Here's how the part is built. I have some questions about the finished solid (model axes, mm). Round coordinates to 2 decimals unless told otherwise and drop trailing zeros. Order: outer loops, then holes, each group sorted by start corner. A loop starts at its lowest first (then second) coordinate and runs counter-clockwise, first axis right, second up. Notation, with made-up numbers: (2.25, 84) - (47.25, 84) arc R18 ccw to (47.25, 102) - close; hole circle Ø11 at (-29.75, 62). An arc over 180 degrees is marked (long way). One line per item, written item: value.
from build123d import *

# Parameters (mm, degrees)
SKETCH1_R           = 2.4892
SKETCH1_R_2         = 14.2875
SKETCH1_R_3         = 9.525
BOSS_EXTRUDE1_DEPTH = 3.175
FILLET1_R           = 10.16


with BuildPart() as part:
    # Sketch1 → Boss-Extrude1 (new body)
    with BuildSketch(Plane.XY):
        Polygon((0, 0), (304.8, 0), (304.8, 116.084254136), (286.959727495, 165.1), (0, 165.1), align=None)
        with Locations((12.7, 158.75)):
            Circle(SKETCH1_R, mode=Mode.SUBTRACT)
        with Locations((38.1, 6.35)):
            Circle(SKETCH1_R, mode=Mode.SUBTRACT)
        with Locations((25.4, 158.75)):
            Circle(SKETCH1_R, mode=Mode.SUBTRACT)
        with Locations((38.1, 158.75)):
            Circle(SKETCH1_R, mode=Mode.SUBTRACT)
        with Locations((25.4, 146.05)):
            Circle(SKETCH1_R, mode=Mode.SUBTRACT)
        with Locations((38.1, 146.05)):
            Circle(SKETCH1_R, mode=Mode.SUBTRACT)
        with Locations((25.4, 133.35)):
            Circle(SKETCH1_R, mode=Mode.SUBTRACT)
        with Locations((38.1, 133.35)):
            Circle(SKETCH1_R, mode=Mode.SUBTRACT)
        with Locations((25.4, 120.65)):
            Circle(SKETCH1_R, mode=Mode.SUBTRACT)
        with Locations((38.1, 120.65)):
            Circle(SKETCH1_R, mode=Mode.SUBTRACT)
        with Locations((25.4, 107.95)):
            Circle(SKETCH1_R, mode=Mode.SUBTRACT)
        with Locations((38.1, 107.95)):
            Circle(SKETCH1_R, mode=Mode.SUBTRACT)
        with Locations((25.4, 95.25)):
            Circle(SKETCH1_R, mode=Mode.SUBTRACT)
        with Locations((38.1, 95.25)):
            Circle(SKETCH1_R, mode=Mode.SUBTRACT)
        with Locations((25.4, 82.55)):
            Circle(SKETCH1_R, mode=Mode.SUBTRACT)
        with Locations((38.1, 82.55)):
            Circle(SKETCH1_R, mode=Mode.SUBTRACT)
        with Locations((25.4, 69.85)):
            Circle(SKETCH1_R, mode=Mode.SUBTRACT)
        with Locations((38.1, 69.85)):
            Circle(SKETCH1_R, mode=Mode.SUBTRACT)
        with Locations((25.4, 57.15)):
            Circle(SKETCH1_R, mode=Mode.SUBTRACT)
        with Locations((38.1, 57.15)):
            Circle(SKETCH1_R, mode=Mode.SUBTRACT)
        with Locations((25.4, 44.45)):
            Circle(SKETCH1_R, mode=Mode.SUBTRACT)
        with Locations((38.1, 44.45)):
            Circle(SKETCH1_R, mode=Mode.SUBTRACT)
        with Locations((25.4, 31.75)):
            Circle(SKETCH1_R, mode=Mode.SUBTRACT)
        with Locations((38.1, 31.75)):
            Circle(SKETCH1_R, mode=Mode.SUBTRACT)
        with Locations((25.4, 19.05)):
            Circle(SKETCH1_R, mode=Mode.SUBTRACT)
        with Locations((38.1, 19.05)):
            Circle(SKETCH1_R, mode=Mode.SUBTRACT)
        with Locations((25.4, 6.35)):
            Circle(SKETCH1_R, mode=Mode.SUBTRACT)
        with Locations((12.7, 146.05)):
            Circle(SKETCH1_R, mode=Mode.SUBTRACT)
        with Locations((12.7, 133.35)):
            Circle(SKETCH1_R, mode=Mode.SUBTRACT)
        with Locations((12.7, 120.65)):
            Circle(SKETCH1_R, mode=Mode.SUBTRACT)
        with Locations((12.7, 107.95)):
            Circle(SKETCH1_R, mode=Mode.SUBTRACT)
        with Locations((12.7, 95.25)):
            Circle(SKETCH1_R, mode=Mode.SUBTRACT)
        with Locations((12.7, 82.55)):
            Circle(SKETCH1_R, mode=Mode.SUBTRACT)
        with Locations((12.7, 69.85)):
            Circle(SKETCH1_R, mode=Mode.SUBTRACT)
        with Locations((12.7, 57.15)):
            Circle(SKETCH1_R, mode=Mode.SUBTRACT)
        with Locations((12.7, 44.45)):
            Circle(SKETCH1_R, mode=Mode.SUBTRACT)
        with Locations((12.7, 31.75)):
            Circle(SKETCH1_R, mode=Mode.SUBTRACT)
        with Locations((12.7, 19.05)):
            Circle(SKETCH1_R, mode=Mode.SUBTRACT)
        with Locations((12.7, 6.35)):
            Circle(SKETCH1_R, mode=Mode.SUBTRACT)
        with Locations((248.678017777, 158.881185382)):
            Circle(SKETCH1_R, mode=Mode.SUBTRACT)
        with Locations((264.955769881, 151.290744918)):
            Circle(SKETCH1_R, mode=Mode.SUBTRACT)
        with Locations((276.889866165, 155.634400739)):
            Circle(SKETCH1_R, mode=Mode.SUBTRACT)
        with Locations((253.021673597, 146.947089098)):
            Circle(SKETCH1_R, mode=Mode.SUBTRACT)
        with Locations((269.299425702, 139.356648634)):
            Circle(SKETCH1_R, mode=Mode.SUBTRACT)
        with Locations((281.233521986, 143.700304455)):
            Circle(SKETCH1_R, mode=Mode.SUBTRACT)
        with Locations((257.365329418, 135.012992814)):
            Circle(SKETCH1_R, mode=Mode.SUBTRACT)
        with Locations((273.643081522, 127.42255235)):
            Circle(SKETCH1_R, mode=Mode.SUBTRACT)
        with Locations((285.577177806, 131.766208171)):
            Circle(SKETCH1_R, mode=Mode.SUBTRACT)
        with Locations((261.708985238, 123.07889653)):
            Circle(SKETCH1_R, mode=Mode.SUBTRACT)
        with Locations((277.986737342, 115.488456066)):
            Circle(SKETCH1_R, mode=Mode.SUBTRACT)
        with Locations((289.920833626, 119.832111887)):
            Circle(SKETCH1_R, mode=Mode.SUBTRACT)
        with Locations((266.052641058, 111.144800246)):
            Circle(SKETCH1_R, mode=Mode.SUBTRACT)
        with Locations((282.330393162, 103.554359782)):
            Circle(SKETCH1_R, mode=Mode.SUBTRACT)
        with Locations((294.264489446, 107.898015603)):
            Circle(SKETCH1_R, mode=Mode.SUBTRACT)
        with Locations((270.396296878, 99.210703962)):
            Circle(SKETCH1_R, mode=Mode.SUBTRACT)
        with Locations((279.4, 69.85)):
            Circle(SKETCH1_R, mode=Mode.SUBTRACT)
        with Locations((266.7, 69.85)):
            Circle(SKETCH1_R, mode=Mode.SUBTRACT)
        with Locations((292.1, 69.85)):
            Circle(SKETCH1_R, mode=Mode.SUBTRACT)
        with Locations((266.7, 57.15)):
            Circle(SKETCH1_R, mode=Mode.SUBTRACT)
        with Locations((279.4, 57.15)):
            Circle(SKETCH1_R, mode=Mode.SUBTRACT)
        with Locations((292.1, 57.15)):
            Circle(SKETCH1_R, mode=Mode.SUBTRACT)
        with Locations((266.7, 44.45)):
            Circle(SKETCH1_R, mode=Mode.SUBTRACT)
        with Locations((279.4, 44.45)):
            Circle(SKETCH1_R, mode=Mode.SUBTRACT)
        with Locations((292.1, 44.45)):
            Circle(SKETCH1_R, mode=Mode.SUBTRACT)
        with Locations((266.7, 31.75)):
            Circle(SKETCH1_R, mode=Mode.SUBTRACT)
        with Locations((279.4, 31.75)):
            Circle(SKETCH1_R, mode=Mode.SUBTRACT)
        with Locations((292.1, 31.75)):
            Circle(SKETCH1_R, mode=Mode.SUBTRACT)
        with Locations((266.7, 19.05)):
            Circle(SKETCH1_R, mode=Mode.SUBTRACT)
        with Locations((279.4, 19.05)):
            Circle(SKETCH1_R, mode=Mode.SUBTRACT)
        with Locations((292.1, 19.05)):
            Circle(SKETCH1_R, mode=Mode.SUBTRACT)
        with Locations((266.7, 6.35)):
            Circle(SKETCH1_R, mode=Mode.SUBTRACT)
        with Locations((279.4, 6.35)):
            Circle(SKETCH1_R, mode=Mode.SUBTRACT)
        with Locations((292.1, 6.35)):
            Circle(SKETCH1_R, mode=Mode.SUBTRACT)
        with Locations((117.275545981, 66.937360953)):
            Circle(SKETCH1_R_2, mode=Mode.SUBTRACT)
        with Locations((167.147605731, 115.915231493)):
            Circle(SKETCH1_R_2, mode=Mode.SUBTRACT)
        with Locations((169.269677971, 55.177793896)):
            Circle(SKETCH1_R_2, mode=Mode.SUBTRACT)
        with Locations((215.081758022, 82.498279276)):
            Circle(SKETCH1_R_2, mode=Mode.SUBTRACT)
        with Locations((87.96680696, 101.664655725)):
            Circle(SKETCH1_R_3, mode=Mode.SUBTRACT)
        with Locations((87.96680696, 32.068655725)):
            Circle(SKETCH1_R_3, mode=Mode.SUBTRACT)
        with Locations((87.96680696, 127.064655725)):
            Circle(SKETCH1_R, mode=Mode.SUBTRACT)
        with Locations((109.963852217, 114.364655725)):
            Circle(SKETCH1_R, mode=Mode.SUBTRACT)
        with Locations((109.963852217, 88.964655725)):
            Circle(SKETCH1_R, mode=Mode.SUBTRACT)
        with Locations((87.96680696, 76.264655725)):
            Circle(SKETCH1_R, mode=Mode.SUBTRACT)
        with Locations((65.969761704, 88.964655725)):
            Circle(SKETCH1_R, mode=Mode.SUBTRACT)
        with Locations((65.969761704, 114.364655725)):
            Circle(SKETCH1_R, mode=Mode.SUBTRACT)
        with Locations((87.96680696, 6.668655725)):
            Circle(SKETCH1_R, mode=Mode.SUBTRACT)
        with Locations((65.969761704, 19.368655725)):
            Circle(SKETCH1_R, mode=Mode.SUBTRACT)
        with Locations((65.969761704, 44.768655725)):
            Circle(SKETCH1_R, mode=Mode.SUBTRACT)
        with Locations((87.96680696, 57.468655725)):
            Circle(SKETCH1_R, mode=Mode.SUBTRACT)
        with Locations((109.963852217, 44.768655725)):
            Circle(SKETCH1_R, mode=Mode.SUBTRACT)
        with Locations((109.963852217, 19.368655725)):
            Circle(SKETCH1_R, mode=Mode.SUBTRACT)
    extrude(amount=BOSS_EXTRUDE1_DEPTH)

    # Fillet1
    fillet1_edges = [part.edges().sort_by_distance(p)[0] for p in [
        (286.959727495, 165.1, 1.5875),
        (304.8, 116.084254136, 1.5875),
        (304.8, 0, 1.5875),
        (0, 0, 1.5875),
        (0, 165.1, 1.5875),
    ]]
    fillet(fillet1_edges, radius=FILLET1_R)


solid = part.part
Q1. If we section it at C-C, the plane z = 0.9: Give the number of separate pieces and of enclosed holes in the cut face, then the cut area to 3 significant figures.
Results list:
separate pieces: 1
enclosed holes: 91
area: 45,000 mm²
Q2. If we section it at B-B, the plane x = 224.5: Please give me the cut outline in (y, z) (3 decimals).
Results list:
outline: (0, 0) - (71.754, 0) - (71.754, 3.175) - (0, 3.175) - close; (93.242, 0) - (165.1, 0) - (165.1, 3.175) - (93.242, 3.175) - close
Q3. If we section it at A-A, the plane x = 126: Please give me the cut outline in (y, z) (3 decimals).
Results list:
outline: (0, 0) - (55.623, 0) - (55.623, 3.175) - (0, 3.175) - close; (78.252, 0) - (165.1, 0) - (165.1, 3.175) - (78.252, 3.175) - close
Q4. If I drill on line 1 along X through (y, z) = (79, 1.8); line 2 along X through (y, z) = (144, 1.6); line 3 along Y through (x, z) = (84.5, 1.4), over which ranges is the centre line in solid material (lowest first)?
Results list:
line 1: 0 to 109.62, 124.93 to 201.23, 228.93 to 304.8
line 2: 0 to 11.29, 14.11 to 23.99, 26.81 to 36.69, 39.51 to 278.76, 283.7 to 294.64
line 3: 0 to 23.2, 40.94 to 92.79, 110.54 to 165.1
Q5. We'd pull the mould along X, two halves only. Please class faces 1 (the cylindrical face through (78.45, 32.49, 1.57)), 2 (the cylindrical face through (3.055, 2.897, 1.61)), 3 (the cylindrical face through (285.602, 163.312, 1.61)): released by +X, released by -X, zero draft, split by the parting line, or undercut.
Results list:
face 1: undercut
face 2: released by -X
face 3: released by +X
